Part model, mm, in its own coordinate system. Give positions to 0.01 mm unless a question says otherwise; leave off trailing zeros. Write each loop counter-clockwise with the first axis right and the second up, starting at its lowest first coordinate (ties: lowest second). Pieces come first, ordered by that corner, then holes.
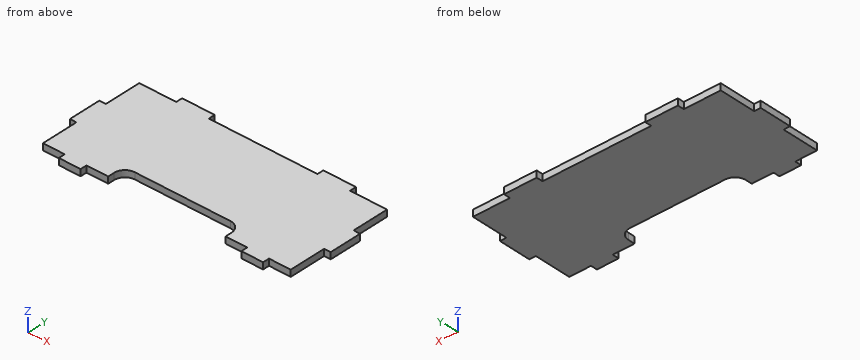
from build123d import *

# Parameters (mm, degrees)
BOSS_EXTRUDE1_DEPTH = 3


with BuildPart() as part:
    # Sketch1 → Boss-Extrude1 (new body)
    with BuildSketch(Plane.XY):
        with BuildLine():
            Line((-57, -28.5), (-57, -11.5))
            Line((-57, -11.5), (-60, -11.5))
            Line((-60, -11.5), (-60, 3.5))
            Line((-60, 3.5), (-57, 3.5))
            Line((-57, 3.5), (-57, 20.5))
            Line((-57, 20.5), (-40, 20.5))
            Line((-40, 20.5), (-40, 23.5))
            Line((-40, 23.5), (-25, 23.5))
            Line((-25, 23.5), (-25, 20.5))
            Line((-25, 20.5), (25, 20.5))
            Line((25, 20.5), (25, 23.5))
            Line((25, 23.5), (40, 23.5))
            Line((40, 23.5), (40, 20.5))
            Line((40, 20.5), (57, 20.5))
            Line((57, 20.5), (57, 3.5))
            Line((57, 3.5), (60, 3.5))
            Line((60, 3.5), (60, -11.5))
            Line((60, -11.5), (57, -11.5))
            Line((57, -11.5), (57, -28.5))
            Line((57, -28.5), (47, -28.5))
            Line((47, -28.5), (47, -31.5))
            Line((47, -31.5), (37, -31.5))
            Line((37, -31.5), (37, -28.5))
            Line((37, -28.5), (27, -28.5))
            Line((27, -28.5), (27, -25.5))
            ThreePointArc((27, -25.5), (25.535533906, -21.964466094), (22, -20.5))
            Line((22, -20.5), (-22, -20.5))
            ThreePointArc((-22, -20.5), (-25.535533906, -21.964466094), (-27, -25.5))
            Line((-27, -25.5), (-27, -28.5))
            Line((-27, -28.5), (-37, -28.5))
            Line((-37, -28.5), (-37, -31.5))
            Line((-37, -31.5), (-47, -31.5))
            Line((-47, -31.5), (-47, -28.5))
            Line((-47, -28.5), (-57, -28.5))
        make_face()
    extrude(amount=BOSS_EXTRUDE1_DEPTH)


solid = part.part
1) Saw through at B-B (x = 44.5). Write the cut outline in (y, z).
Check result:
outline: (-31.5, 0) - (20.5, 0) - (20.5, 3) - (-31.5, 3) - close
2) Flat gauge pins, fed straight in: P1, Ø0.9, axis at y = -26.5, z = 2, coming from the +X side; P2, Ø0.9, axis at x = 34, z = 2, coming from the -Y side; P3, Ø1.5, axis at x = 59, z = 1, coming from the +Y side. Where does each tip first touch, or does it go through?
Check result:
P1: stops at x = 57
P2: stops at y = -28.5
P3: stops at y = 3.5
3) Saw through at C-C (y = 10.5). Write the cut outline in (x, z).
Check result:
outline: (-57, 0) - (57, 0) - (57, 3) - (-57, 3) - close
4) Drill centre lines: L1, parallel to X at y = -29, z = 1.8; L2, parallel to X at y = 21, z = 1.35; L3, parallel to Y at x = 22.5, z = 1. Where is each one in solid material? Low to high.
Check result:
L1: x = -47 to -37, 37 to 47
L2: x = -40 to -25, 25 to 40
L3: y = -20.53 to 20.5
